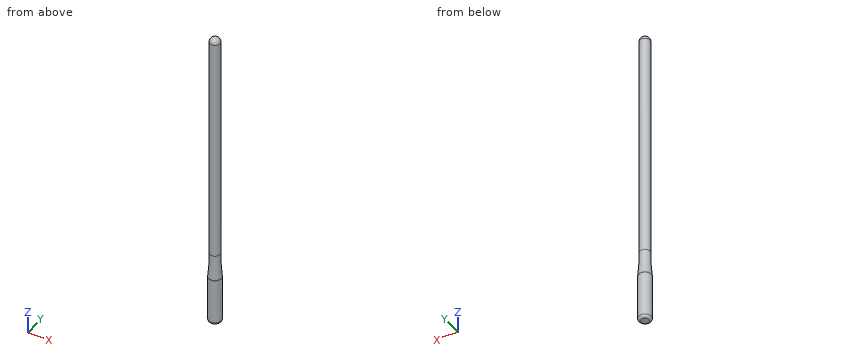
from build123d import *

# Parameters (mm, degrees)
F0_R     = 2.54
F1_DEPTH = 152.4
F2_R     = 2.54
F0_R_2   = 3.175
F3_DEPTH = 25.4
F5_R     = 127
F6_R     = 1.27


# Not quite as in the source:
# - a fillet or chamfer that OpenCascade refuses, or shapes differently, is made with other operations: its cross-section is extruded or revolved along the edge and cut away or added


with BuildPart() as f1:
    # F0 (on Top) → F1 (new body)
    with BuildSketch(Plane.XY):
        Circle(F0_R)
    extrude(amount=F1_DEPTH)

    # F2
    f2_edges = [f1.edges().sort_by_distance(p)[0] for p in [
        (-2.54, 0, 152.4),
    ]]
    fillet(f2_edges, radius=F2_R)

    # F0 (on Top) → F3 (join)
    with BuildSketch(Plane.XY):
        Circle(F0_R_2)
        Circle(F0_R, mode=Mode.SUBTRACT)
    extrude(amount=F3_DEPTH)

    # F4: fillet of radius 2.54 on 1 edges, made by hand

    # F4_s1 → F4_t2 (revolve, cut)
    with BuildSketch(Plane.XZ):
        with BuildLine():
            ThreePointArc((2.54, 25.4), (3.0109524406, 24.6179735296), (3.175, 23.7199479175))
            Line((3.175, 23.7199479175), (3.175, 25.4))
            Line((3.175, 25.4), (2.54, 25.4))
        make_face()
    revolve(axis=Axis((0, 0, 25.4), (0, 0, 1)), mode=Mode.SUBTRACT)

    # F5
    f5_edges = [f1.edges().sort_by_distance(p)[0] for p in [
        (-2.54, 0, 25.4),
    ]]
    fillet(f5_edges, radius=F5_R)

    # F6
    f6_edges = [f1.edges().sort_by_distance(p)[0] for p in [
        (-3.175, 0, 0),
    ]]
    fillet(f6_edges, radius=F6_R)


solid = f1.part
Read the model definition and answer for the solid it produces. Units are mm, in the model's axes. Round coordinates to 2 decimals unless told otherwise and drop trailing zeros. Write each loop counter-clockwise with the first axis right and the second up, starting at its lowest first coordinate (ties: lowest second). Pieces come first, ordered by that corner, then holes. Notation, with made-up numbers: (32.25, -33) - (63.25, -33) arc R16 cw to (63.25, -8) - close; hole circle Ø6 at (-27.5, 66). An arc over 180 degrees is marked (long way). One line per question, with ' | ' between items. Start each with the question number.
1. Each of these flat-tipped pins is pushed along its axis until it touches: pin 1 (1.5 mm diameter, centred on x = 0, z = 71, fed in from -Y); pin 2 (1 mm diameter, centred on y = 2, z = 121.5, fed in from -X); pin 3 (2 mm diameter, centred on y = 2, z = 123.5, fed in from -X). Where does it stop, or does it pass through?
2. Section A-A (z = 142.5) is taken. Determine the outline of the cut face in (x, y).
3. Find the intervals of material crossed by probe 1 along X at (y, z) = (0.25, 39); probe 2 along X at (y, z) = (1.5, 94.5), in increasing order. Write a range as [from, to].
Filled in:
1) pin 1: y = -2.54 | pin 2: x = -2.05 | pin 3: x = -2.33
2) outline: circle Ø5.08 at (0, 0)
3) probe 1: [-2.53, 2.53] | probe 2: [-2.05, 2.05]
